Work out the finished part from the listing and answer in its coordinate system (mm). A direction names the side the tool comes from. Coordinates: 2 decimals unless noted, no trailing zeros. Order: outer loops, then holes, each group sorted by start corner. A loop starts at its lowest first (then second) coordinate and runs counter-clockwise, first axis right, second up. Notation, with made-up numbers: (-38.75, 1) -> (-16.75, 1) arc R15 ccw to (-16.75, 11) -> close; hole circle Ø3 at (48, 13.5). An arc over 180 degrees is marked (long way). Use one line per item in the form item = value.
from build123d import *

# Parameters (mm, degrees)
CYLINDER018_R          = 4.1
CYLINDER018_DEPTH      = 10
CYLINDER018_ROLL_ANGLE = 90
CYLINDER016_R          = 10.55
CYLINDER016_DEPTH      = 10
CYLINDER016_ROLL_ANGLE = 90
PAD_DEPTH              = 25
FILLET004_R            = 12


with BuildPart() as cilindro018:
    # Cylinder018 → Cylinder018 (new body)
    with BuildSketch(Plane.XY):
        Circle(CYLINDER018_R)
    extrude(amount=CYLINDER018_DEPTH)


with BuildPart() as cilindro018_1:
    # Cylinder018 roll: moved
    add(cilindro018.part.rotate(Axis((0, 0, 0), (1, 0, 0)), CYLINDER018_ROLL_ANGLE))


with BuildPart() as cilindro018_2:
    # Cylinder018 placement: moved
    add(cilindro018_1.part.moved(Location((0, -14, 0))))


with BuildPart() as obj1:
    # Cylinder016 → Cylinder016 (new body)
    with BuildSketch(Plane.XY):
        Circle(CYLINDER016_R)
    extrude(amount=CYLINDER016_DEPTH)


with BuildPart() as obj1_1:
    # Cylinder016 roll: moved
    add(obj1.part.rotate(Axis((0, 0, 0), (1, 0, 0)), CYLINDER016_ROLL_ANGLE))


with BuildPart() as obj1_2:
    # Cylinder016 placement: moved
    add(obj1_1.part.moved(Location((0, -22.5, 0))))

    # Fusion001: union Cilindro018
    add(cilindro018_2.part)


with BuildPart() as cut023003:
    # Sketch → Pad (new body)
    with BuildSketch(Plane.XY):
        with BuildLine():
            Line((-25, -30), (-25, -25))
            Line((-25, -25), (35, -25))
            ThreePointArc((35, -25), (42.071068, -22.071068), (45, -15))
            Line((45, -15), (45, 10))
            ThreePointArc((45, 10), (42.071068, 17.071068), (35, 20))
            Line((35, 20), (-25, 20))
            Line((-25, 20), (-25, 25))
            Line((-25, 25), (125, 25))
            Line((125, 25), (125, 20))
            Line((125, 20), (65, 20))
            ThreePointArc((65, 20), (57.928932, 17.071068), (55, 10))
            Line((55, 10), (55, -15))
            ThreePointArc((55, -15), (57.928932, -22.071068), (65, -25))
            Line((65, -25), (125, -25))
            Line((125, -25), (125, -30))
            Line((125, -30), (-25, -30))
        make_face()
    extrude(amount=PAD_DEPTH)

    # Fillet004
    fillet004_edges = [cut023003.edges().sort_by_distance(p)[0] for p in [
        (-25, -27.5, 0),
        (-25, -27.5, 25),
        (-25, 22.5, 0),
        (-25, 22.5, 25),
        (125, 22.5, 0),
        (125, 22.5, 25),
        (125, -27.5, 0),
        (125, -27.5, 25),
    ]]
    fillet(fillet004_edges, radius=FILLET004_R)


with BuildPart() as cut023003_1:
    # Fillet004 placement: moved
    add(cut023003.part.moved(Location((9.841811, 4.997794, -12.933897))))

    # Cut023003: cut obj1
    add(obj1_2.part, mode=Mode.SUBTRACT)


solid = cut023003_1.part
(1) Each of these flat-tipped pins is pushed along its axis until it touches: P1, Ø3, axis at y = -7, z = -1.5, coming from the +X side; P2, Ø5, axis at x = 0, z = 0, coming from the -Y side; P3, Ø3, axis at y = -9.5, z = -6.5, coming from the +X side. Where does it stop, or does it pass through?
Data:
P1 = 64.84
P2 = 25
P3 = 64.89
(2) Section A-A on x = 0 is taken. Write down the section's boundary in (y, z).
Data:
outline = (-25, -12.93) -> (-20, -12.93) -> (-20, -4.1) -> (-22.5, -4.1) -> (-22.5, -10.55) -> (-25, -10.55) -> close; (-25, 10.55) -> (-22.5, 10.55) -> (-22.5, 4.1) -> (-20, 4.1) -> (-20, 12.07) -> (-25, 12.07) -> close; (25, -12.93) -> (30, -12.93) -> (30, 12.07) -> (25, 12.07) -> close
(3) Straight lines are drawn through the part: line 1 along Y through (x, z) = (9, -0.75); line 2 along Z through (x, y) = (0, -21.5); line 3 along Y through (x, z) = (42, 1.5). For each, find the intervals that lie inside material, in ascending order.
Data:
line_1 = -22.5 to -20, 25 to 30
line_2 = -12.93 to -4.1, 4.1 to 12.07
line_3 = -25 to -20, 25 to 30
(4) Which of the six approach directions +Z, -Z, +X, -X, +Y, -Y give full straight-line access (tool end or side, diameter ignored) to faces 4 (the cylindrical face through (131.42, -22.537, -9.325)), 5 (the flat face through (64.842, 3, -1)), 6 (the cylindrical face through (-0.534, -21.234, 4.065)), 7 (the flat face through (15, 24.998, -1))?
Data:
face_4 = -Z, +X, +Y, -Y
face_5 = +Z, -Z, +X
face_6 = -Y
face_7 = +Z, -Z, -X
(5) Section D-D on y = -2.5 is taken. Write down the section's boundary in (x, z), plus the area to 3 significant figures.
Data:
outline = (54.84, -12.93) -> (64.84, -12.93) -> (64.84, 12.07) -> (54.84, 12.07) -> close
area = 250 mm²
(6) The mould has two halves that part along X. Classify faces 1 (the flat face through (105, 24.998, -1)), 2 (the flat face through (5, -22.5, 0)), 3 (the cylindrical face through (131.42, 27.463, -9.325)): released by +X, released by -X, zero draft, split by the parting line, or undercut.
Data:
face_1 = zero draft
face_2 = undercut
face_3 = released by +X
(7) Section B-B on x = 33 is taken. Write down the section's boundary in (y, z), plus the area to 3 significant figures.
Data:
outline = (-25, -12.93) -> (-20, -12.93) -> (-20, 12.07) -> (-25, 12.07) -> close; (25, -12.93) -> (30, -12.93) -> (30, 12.07) -> (25, 12.07) -> close
area = 250 mm²
(8) Section C-C on z = -8.75 is taken. Write down the section's boundary in (x, y).
Data:
outline = (-12.26, -25) -> (-5.89, -25) -> (-5.89, -22.5) -> (5.89, -22.5) -> (5.89, -25) -> (131.95, -25) -> (131.95, -20) -> (74.84, -20) arc R10 cw to (64.84, -10) -> (64.84, 15) arc R10 cw to (74.84, 25) -> (131.95, 25) -> (131.95, 30) -> (-12.26, 30) -> (-12.26, 25) -> (44.84, 25) arc R10 cw to (54.84, 15) -> (54.84, -10) arc R10 cw to (44.84, -20) -> (-12.26, -20) -> close
